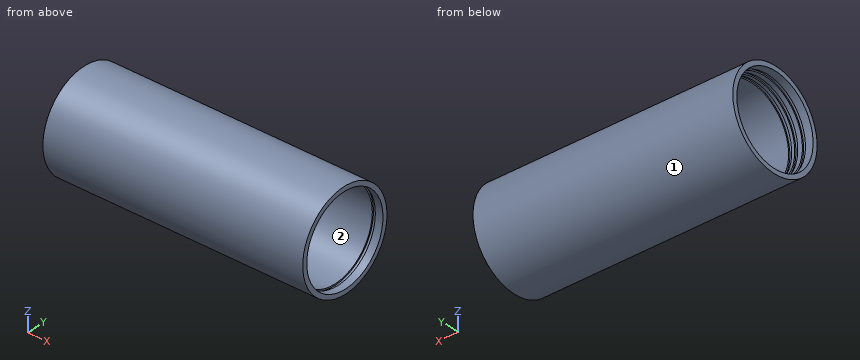
Autodesk Fusion 360 part; units mm, degrees
sketch "Sketch1" plane through (0, 0, 0) normal (1, 0, 0) x (0, 1, 0)
  circle A0 centre (0, 0) radius 28.6
  circle A1 centre (0, 0) radius 31.6
  dimension "d9" = 57.2
  dimension "d10" = 63.2
extrude "Extrude1" add sketch "Sketch1" along normal blind 170
ref_plane "WorkPlane1" through (5, 0, 0) normal (1, 0, 0) x (0, 1, 0)
sketch "Sketch2" plane through (5, 0, 0) normal (1, 0, 0) x (0, 1, 0)
  circle A0 centre (0, 0) radius 29.5
  dimension "d14" = 59
extrude "Extrude2" cut sketch "Sketch2" along normal blind 2
ref_plane "WorkPlane2" through (165, 0, 0) normal (1, 0, 0) x (0, 1, 0)
sketch "Sketch3" plane through (165, 0, 0) normal (1, 0, 0) x (0, 1, 0)
  circle A0 centre (0, 0) radius 29.5
  dimension "d18" = 59
extrude "Extrude3" cut sketch "Sketch3" against normal blind 2
sketch "Sketch4" plane through (0, 0, 0) normal (1, 0, 0) x (0, 1, 0)
ref_plane "WorkPlane4" through (0, 0, 0) normal (1, 0, 0) x (0, 1, 0)
ref_plane "WorkPlane5" through (10, 0, 0) normal (1, 0, 0) x (0, 1, 0)
sketch "Sketch5" plane through (10, 0, 0) normal (1, 0, 0) x (0, 1, 0)
  circle A0 centre (0, 0) radius 29.5
  dimension "d24" = 59
extrude "Extrude4" cut sketch "Sketch5" along normal blind 2
ref_plane "WorkPlane6" through (14, 0, 0) normal (1, 0, 0) x (0, 1, 0)
sketch "Sketch6" plane through (14, 0, 0) normal (1, 0, 0) x (0, 1, 0)
  circle A0 centre (0, 0) radius 29.5
  dimension "d28" = 59
extrude "Extrude5" cut sketch "Sketch6" along normal blind 2
Geometry: final body of the model. Coordinates: model frame, mm. Face numbers are marked on the shaded views. Coordinates: 2 decimals unless noted, no trailing zeros. Loops run counter-clockwise (first coordinate to the right, second up) from the corner with the lowest first, then second, coordinate; pieces in that order, holes last. Notation, with made-up numbers: M 37,0 L 56,0 A13 ccw 56,5 Z; hole C 19,69 d8. An arc over 180 degrees is marked long. One line per item, written item: value. Start each with the question number.
1) Pin query (flat end, axial travel): P1, Ø1.5, axis at x = 137, y = -19, coming from the +Z side; P2, Ø10, axis at x = 139, z = -12.5, coming from the +Y side; P3, Ø6, axis at x = 53.5, z = 20, coming from the +Y side; P4, Ø12, axis at y = 17.5, z = -20.5, coming from the -X side. Return the tip coordinate at first contact, or that it passes through.
2) Cut plane A-A (x = 89). Return loops of the section in (y, z), then the cut area to 3 significant figures.
3) Draft query along Y for the marked faces 1 and 2. Return one class per face: released by +Y, released by -Y, zero draft, split by the parting line, or undercut.
4) Material intervals for L1, parallel to Z at x = 15.45, y = 0; L2, parallel to Z at x = 50, y = -22.5; L3, parallel to Y at x = 123.5, z = -8.5, sorted ascending. Write a range as from..to.
Evaluation:
1. P1: z = 25.8
1. P2: y = 30.7
1. P3: y = 26.64
1. P4: x = 0
2. outline: C 0,0 d63.2; hole C 0,0 d57.2
2. area: 567 mm^2
3. face 1: split by the parting line
3. face 2: undercut
4. L1: -31.6..-29.5, 29.5..31.6
4. L2: -22.19..-17.66, 17.66..22.19
4. L3: -30.44..-27.31, 27.31..30.44
